Verification items for the finished model (mm, model axes). Face numbers are marked on the shaded views. A direction names the side the tool comes from. Round coordinates to 2 decimals unless told otherwise and drop trailing zeros. Order: outer loops, then holes, each group sorted by start corner. A loop starts at its lowest first (then second) coordinate and runs counter-clockwise, first axis right, second up. Notation, with made-up numbers: (-23.5, 57.25) -> (13.5, 57.25) arc R12 ccw to (13.5, 80.25) -> close; hole circle Ø10 at (-29.75, 62.25). An arc over 180 degrees is marked (long way). Write item = value, one per line. Start each with the question number.
from build123d import *

# Parameters (mm, degrees)
SKETCH1_R      = 25
EXTRUDE1_DEPTH = 5
SKETCH4_R      = 1.5
EXTRUDE2_DEPTH = 5
SKETCH6_R      = 2.8
EXTRUDE4_DEPTH = 2
SKETCH7_R      = 42.8625
SKETCH7_R_2    = 23.8125
EXTRUDE5_DEPTH = 2


with BuildPart() as part:
    # Sketch1 → Extrude1 (new body)
    with BuildSketch(Plane.XY):
        Circle(SKETCH1_R)
    extrude(amount=EXTRUDE1_DEPTH)

    # Sketch4 → Extrude2 (add)
    with BuildSketch(Plane.XY.offset(5)):
        with BuildLine():
            Line((-13.007376983, 65.393912324), (-4.682070455, 23.538866078))
            ThreePointArc((-4.682070455, 23.538866078), (0, 24), (4.682070455, 23.538866078))
            Line((4.682070455, 23.538866078), (13.007376983, 65.393912324))
            ThreePointArc((13.007376983, 65.393912324), (0, 66.675), (-13.007376983, 65.393912324))
        make_face()
        with Locations((0, 62.675)):
            Circle(SKETCH4_R, mode=Mode.SUBTRACT)
        with BuildLine():
            Line((65.393912324, 13.007376983), (23.538866078, 4.682070455))
            ThreePointArc((23.538866078, 4.682070455), (24, 0), (23.538866078, -4.682070455))
            Line((23.538866078, -4.682070455), (65.393912324, -13.007376983))
            ThreePointArc((65.393912324, -13.007376983), (66.675, 0), (65.393912324, 13.007376983))
        make_face()
        with Locations((62.675, 0)):
            Circle(SKETCH4_R, mode=Mode.SUBTRACT)
        with BuildLine():
            Line((4.682070455, -23.538866078), (13.007376983, -65.393912324))
            ThreePointArc((13.007376983, -65.393912324), (0, -66.675), (-13.007376983, -65.393912324))
            Line((-13.007376983, -65.393912324), (-4.682070455, -23.538866078))
            ThreePointArc((-4.682070455, -23.538866078), (0, -24), (4.682070455, -23.538866078))
        make_face()
        with Locations((0, -62.675)):
            Circle(SKETCH4_R, mode=Mode.SUBTRACT)
        with BuildLine():
            Line((-23.538866078, -4.682070455), (-65.393912324, -13.007376983))
            ThreePointArc((-65.393912324, -13.007376983), (-66.675, 0), (-65.393912324, 13.007376983))
            Line((-65.393912324, 13.007376983), (-23.538866078, 4.682070455))
            ThreePointArc((-23.538866078, 4.682070455), (-24, 0), (-23.538866078, -4.682070455))
        make_face()
        with Locations((-62.675, 0)):
            Circle(SKETCH4_R, mode=Mode.SUBTRACT)
    extrude(amount=-EXTRUDE2_DEPTH)

    # Sketch6 → Extrude4 (add)
    with BuildSketch(Plane.XY.offset(5)):
        with Locations((-7.9375, -11.1125)):
            Circle(SKETCH6_R)
        with Locations((7.9375, -11.1125)):
            Circle(SKETCH6_R)
        with Locations((0, 12.7)):
            Circle(SKETCH6_R)
    extrude(amount=EXTRUDE4_DEPTH)

    # Sketch7 → Extrude5 (add)
    with BuildSketch(Plane.XY.offset(5)):
        Circle(SKETCH7_R)
        Circle(SKETCH7_R_2, mode=Mode.SUBTRACT)
    extrude(amount=-EXTRUDE5_DEPTH)


solid = part.part
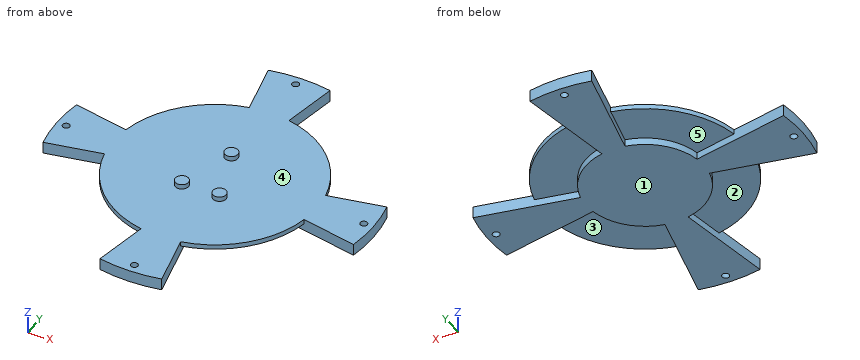
(1) Set-up check for the marked faces 1 and 2: record each of +Z, -Z, +X, -X, +Y, -Y from which the full face is reachable in a straight line by a thin tool's end or side.
(2) Cross-section at D-D (y = 46.5). Enter the section's corners in (x, z).
(3) Scan lines: line 1 along Z through (x, y) = (-9, -6); line 2 along Z through (x, y) = (30.5, 24); line 3 along X through (y, z) = (21.5, 2.25). Record each from-to range of solid material in increasing order. Write a range as from..to.
(4) Depth check by flat-ended pin: pin 1 (3 mm diameter, centred on y = -31, z = 6, fed in from -X); pin 2 (5 mm diameter, centred on x = 62.675, y = 0, fed in from +Z); pin 3 (3 mm diameter, centred on y = -40.5, z = 4, fed in from +X); pin 4 (4 mm diameter, centred on x = 9.5, y = 53, fed in from -Z). Enter the tip coordinate at first touch or a pass-through.
(5) Cross-section at C-C (y = 31). Enter the section's corners in (x, z).
(6) Draft check along Y on the marked faces 3, 4 and 5. Enter one of: +Y half, -Y half, draft (parallel to the pull), parting line (faces both ways), or undercut.
(7) Cross-section at B-B (x = -22.5). Enter the section's corners in (y, z).
(8) Cross-section at A-A (z = 1.5). Enter the section's corners in (x, y) (3 decimals).
Outcome:
q1.face_1 = -Z, +X, -X, +Y, -Y
q1.face_2 = -Z
q2.outline = (-9.25, 0) -> (9.25, 0) -> (9.25, 5) -> (-9.25, 5) -> close
q3.line_1 = 0..5
q3.line_2 = 3..5
q3.line_3 = -12.76..12.76
q4.pin_1 = -30.73
q4.pin_2 = 5
q4.pin_3 = 17.78
q4.pin_4 = 0
q5.outline = (-29.6, 3) -> (-6.17, 3) -> (-6.17, 0) -> (6.17, 0) -> (6.17, 3) -> (29.6, 3) -> (29.6, 5) -> (-29.6, 5) -> close
q6.face_3 = undercut
q6.face_4 = draft
q6.face_5 = undercut
q7.outline = (-36.48, 3) -> (-10.9, 3) -> (-10.9, 0) -> (10.9, 0) -> (10.9, 3) -> (36.48, 3) -> (36.48, 5) -> (-36.48, 5) -> close
q8.outline = (-65.394, -13.007) -> (-24.52, -4.877) arc R25 ccw to (-4.877, -24.52) -> (-13.007, -65.394) arc R66.675 ccw to (13.007, -65.394) -> (4.877, -24.52) arc R25 ccw to (24.52, -4.877) -> (65.394, -13.007) arc R66.675 ccw to (65.394, 13.007) -> (24.52, 4.877) arc R25 ccw to (4.877, 24.52) -> (13.007, 65.394) arc R66.675 ccw to (-13.007, 65.394) -> (-4.877, 24.52) arc R25 ccw to (-24.52, 4.877) -> (-65.394, 13.007) arc R66.675 ccw to start; hole circle Ø3 at (-62.675, 0); hole circle Ø3 at (0, -62.675); hole circle Ø3 at (0, 62.675); hole circle Ø3 at (62.675, 0)
